from build123d import *

# Parameters (mm, degrees)
SKETCH1_W                 = 34.925
SKETCH1_H                 = 9.525
BOSS_EXTRUDE1_DEPTH       = 7.14375
SKETCH2_W                 = 34.925
SKETCH2_H                 = 11.1125
BOSS_EXTRUDE2_DEPTH       = 2.06375
F_6_CLEARANCE_HOLE1_D     = 3.7973
F_6_CLEARANCE_HOLE1_DEPTH = 9.2075
SKETCH5_R                 = 3.81
CUT_EXTRUDE1_DEPTH        = 3.175


with BuildPart() as part:
    # Sketch1 → Boss-Extrude1 (new body)
    with BuildSketch(Plane.XY):
        with Locations((17.4625, 4.7625)):
            Rectangle(SKETCH1_W, SKETCH1_H)
    extrude(amount=BOSS_EXTRUDE1_DEPTH)

    # Sketch2 → Boss-Extrude2 (add)
    with BuildSketch(Plane.XY.offset(7.14375)):
        with Locations((17.4625, 4.7625)):
            Rectangle(SKETCH2_W, SKETCH2_H)
    extrude(amount=BOSS_EXTRUDE2_DEPTH)

    # #6 Clearance Hole1
    with Locations(Plane.XY.offset(9.2075)):
        with Locations((4.7625, 4.7625), (17.4625, 4.7625), (30.1625, 4.7625)):
            Hole(F_6_CLEARANCE_HOLE1_D / 2, depth=F_6_CLEARANCE_HOLE1_DEPTH)

    # Sketch5 → Cut-Extrude1 (cut)
    with BuildSketch(Plane.XY.offset(9.2075)):
        with Locations((4.7625, 4.7625)):
            Circle(SKETCH5_R)
        with Locations((17.4625, 4.7625)):
            Circle(SKETCH5_R)
        with Locations((30.1625, 4.7625)):
            Circle(SKETCH5_R)
    extrude(amount=-CUT_EXTRUDE1_DEPTH, mode=Mode.SUBTRACT)


solid = part.part
Could you check a few things on this model? Use its own coordinates, in mm. A direction names the side the tool comes from. Give positions to 0.01 mm unless a question says otherwise; leave off trailing zeros. Loops run counter-clockwise (first coordinate to the right, second up) from the corner with the lowest first, then second, coordinate; pieces in that order, holes last. Notation, with made-up numbers: M 40,15.25 L 46,15.25 A28 cw 46,38.25 Z; hole C 55,59 d8. An arc over 180 degrees is marked long. Answer as a JSON object with one key per item and string values.
Q1. Suppose I cut it at D-D, the plane x = 30.5. List the corners of the cut face in (y, z) for me (1 decimal), plus the area to 3 significant figures.
Values found:
{"outline": "M -0.8,7.1 L 0,7.1 L 0,0 L 2.9,0 L 2.9,6 L 1,6 L 1,9.2 L -0.8,9.2 Z; M 6.6,0 L 9.5,0 L 9.5,7.1 L 10.3,7.1 L 10.3,9.2 L 8.6,9.2 L 8.6,6 L 6.6,6 Z", "area": "44.3 mm²"}
Q2. If I drill on probe 1 along X at (y, z) = (1.25, 6.75) (3 decimals); probe 2 along X at (y, z) = (6.5, 1.5) (3 decimals); probe 3 along Y at (x, z) = (21, 3) (3 decimals), over which ranges is the centre line in solid material (lowest first)? Write a range as [from, to].
Values found:
{"probe 1": "x = [0, 3.287], [6.238, 15.987], [18.938, 28.687], [31.638, 34.925]", "probe 2": "x = [0, 3.997], [5.528, 16.697], [18.228, 29.397], [30.928, 34.925]", "probe 3": "y = [0, 9.525]"}
Q3. If we mould it in two halves opening along X, with no side actions, what happens to faces 5 (the cylindrical face through (28.409, 4.035, 2.974)), 6 (the flat face through (17, 7, 0)), 7 (the flat face through (34.925, 5, 5))? For each: pulls with the +X half, pulls with the -X half, needs draft (parallel to the pull), parting line crosses it, or undercut.
Values found:
{"face 5": "undercut", "face 6": "needs draft", "face 7": "pulls with the +X half"}
Q4. For P1, Ø1, axis at x = 13.5, y = 3, coming from the -Z side; P2, Ø2, axis at x = 27.5, z = 5.5, coming from the +Y side (3 decimals); P3, Ø4, axis at x = 3.5, y = 6, coming from the +Z side; P4, Ø3.5, axis at x = 18.5, z = 2, coming from the -Y side, each with a flat end and sliding along its axis, tell me the tip position at first contact or that it passes through.
Values found:
{"P1": "stops at z = 0", "P2": "stops at y = 9.525", "P3": "stops at z = 6.03", "P4": "stops at y = 0"}
Q5. Suppose I cut it at C-C, the plane x = 10.5. List the corners of the cut face in (y, z) for me (1 decimal), plus the area to 3 significant figures.
Values found:
{"outline": "M -0.8,7.1 L 0,7.1 L 0,0 L 9.5,0 L 9.5,7.1 L 10.3,7.1 L 10.3,9.2 L -0.8,9.2 Z", "area": "91.0 mm²"}
Q6. Suppose I cut it at A-A, the plane x = 19. List the corners of the cut face in (y, z) for me (1 decimal), plus the area to 3 significant figures.
Values found:
{"outline": "M -0.8,7.1 L 0,7.1 L 0,0 L 3.6,0 L 3.6,6 L 1.3,6 L 1.3,9.2 L -0.8,9.2 Z; M 5.9,0 L 9.5,0 L 9.5,7.1 L 10.3,7.1 L 10.3,9.2 L 8.2,9.2 L 8.2,6 L 5.9,6 Z", "area": "55.4 mm²"}
Q7. For faces 1 (the cylindrical face through (26.356, 4.93, 7.642)), 2 (the cylindrical face through (19.36, 4.85, 2.97)), 3 (the flat face through (17, 0, 4)), 4 (the flat face through (17, 9.525, 4)), which set-ups out of +Z, -Z, +X, -X, +Y, -Y let a thin tool reach every point of the face, with its end or its side?
Values found:
{"face 1": "+Z", "face 2": "+Z, -Z", "face 3": "-Z, +X, -X, -Y", "face 4": "-Z, +X, -X, +Y"}
Q8. Suppose I cut it at B-B, the plane z = 8. List the corners of the cut face in (x, y) for me (1 decimal), plus the area to 3 significant figures.
Values found:
{"outline": "M 0,-0.8 L 34.9,-0.8 L 34.9,10.3 L 0,10.3 Z; hole C 4.8,4.8 d7.6; hole C 17.5,4.8 d7.6; hole C 30.2,4.8 d7.6", "area": "251 mm²"}
